```python
from build123d import *

# Parameters (mm, degrees)
F0_R     = 1.092901
F1_DEPTH = 8.89


with BuildPart() as f1:
    # F0 (on Top) → F1 (new body)
    with BuildSketch(Plane.XY):
        with BuildLine():
            Line((-10.186511, 17.824513), (-30.872961, 17.824513))
            Line((-30.872961, 17.824513), (-20.463953, -0.204419))
            Line((-20.463953, -0.204419), (-30.484094, -17.781989))
            Line((-30.484094, -17.781989), (-10.188458, -18.002097))
            Line((-10.188458, -18.002097), (0, -35.649025))
            Line((0, -35.649025), (10.061664, -18.221712))
            Line((10.061664, -18.221712), (31.196423, -18.450921))
            Line((31.196423, -18.450921), (20.562876, -0.033079))
            Line((20.562876, -0.033079), (30.872961, 17.824513))
            Line((30.872961, 17.824513), (10.252791, 17.824513))
            Line((10.252791, 17.824513), (1.863466, 32.35525))
            ThreePointArc((1.863466, 32.35525), (1.860641, 34.526342), (-0.018168, 35.614335))
            ThreePointArc((-0.018168, 35.614335), (-0.0318, 35.614328), (-0.045431, 35.614235))
            ThreePointArc((-0.045431, 35.614235), (-1.914248, 34.515979), (-1.907155, 32.348355))
            Line((-1.907155, 32.348355), (-10.186511, 17.824513))
        make_face()
        Polygon((-7.632454, -18.029818), (7.537469, -18.194337), (0, -31.249616), align=None, mode=Mode.SUBTRACT)
        Polygon((-11.478418, -15.767821), (-26.717751, -15.602549), (-19.193953, -2.404124), align=None, mode=Mode.SUBTRACT)
        Polygon((6.609826, -15.96399), (-6.587783, -15.820861), (-5.245977, -12.983611), (5.37023, -12.983611), align=None, mode=Mode.SUBTRACT)
        Polygon((-10.226373, -13.537018), (-16.653953, -2.404124), (-13.604161, -2.404124), (-8.723036, -10.85848), align=None, mode=Mode.SUBTRACT)
        Polygon((13.711111, -2.218881), (16.760902, -2.218881), (10.064189, -13.817929), (8.537635, -11.179605), align=None, mode=Mode.SUBTRACT)
        Polygon((11.33557, -16.015242), (19.300902, -2.218881), (27.366612, -16.1891), align=None, mode=Mode.SUBTRACT)
        Polygon((-19.20203, 2.009275), (-27.062961, 15.624808), (-11.440459, 15.624808), align=None, mode=Mode.SUBTRACT)
        Polygon((-13.832127, 2.009275), (-16.678082, 2.009275), (-10.170459, 13.425103), (-8.705827, 10.888287), align=None, mode=Mode.SUBTRACT)
        with BuildLine():
            Line((-6.75627, 0.938559), (-7.088266, 1.774853))
            ThreePointArc((-7.088266, 1.774853), (-6.149591, 2.138201), (-5.143329, 2.114348))
            ThreePointArc((-5.143329, 2.114348), (-4.684085, 1.931017), (-4.344395, 1.571676))
            ThreePointArc((-4.344395, 1.571676), (-4.154791, 0.893336), (-4.344395, 0.214996))
            ThreePointArc((-4.344395, 0.214996), (-4.846257, -0.463524), (-5.50511, -0.990941))
            Line((-5.50511, -0.990941), (-4.118282, -0.990941))
            Line((-4.118282, -0.990941), (-4.118282, -1.940617))
            Line((-4.118282, -1.940617), (-7.133126, -1.940617))
            Line((-7.133126, -1.940617), (-7.133126, -1.262277))
            ThreePointArc((-7.133126, -1.262277), (-6.428669, -0.65133), (-5.761372, 0))
            ThreePointArc((-5.761372, 0), (-5.521749, 0.287364), (-5.354368, 0.622))
            ThreePointArc((-5.354368, 0.622), (-5.409921, 1.056041), (-5.79152, 1.270191))
            ThreePointArc((-5.79152, 1.270191), (-6.315562, 1.225589), (-6.75627, 0.938559))
        make_face(mode=Mode.SUBTRACT)
        with BuildLine():
            ThreePointArc((-3.600539, 0.402436), (-3.456783, 1.145183), (-3.035859, 1.773803))
            ThreePointArc((-3.035859, 1.773803), (-2.669777, 2.034358), (-2.238135, 2.159219))
            ThreePointArc((-2.238135, 2.159219), (-1.951313, 2.178043), (-1.664491, 2.159219))
            ThreePointArc((-1.664491, 2.159219), (-1.180923, 1.946357), (-0.821952, 1.558686))
            ThreePointArc((-0.821952, 1.558686), (-0.52188, 0.80677), (-0.454462, 0))
            ThreePointArc((-0.454462, 0), (-0.581823, -0.858949), (-1.010179, -1.614281))
            ThreePointArc((-1.010179, -1.614281), (-1.43468, -1.87918), (-1.924424, -1.981771))
            ThreePointArc((-1.924424, -1.981771), (-2.520232, -1.899523), (-3.044822, -1.605318))
            ThreePointArc((-3.044822, -1.605318), (-3.443663, -0.96578), (-3.582613, -0.224987))
            ThreePointArc((-3.582613, -0.224987), (-3.602765, 0.088404), (-3.600539, 0.402436))
        make_face(mode=Mode.SUBTRACT)
        Polygon((-4.867668, 12.983611), (-6.392563, 15.624808), (6.461138, 15.624808), (4.938996, 12.983611), align=None, mode=Mode.SUBTRACT)
        Polygon((-7.662563, 17.824513), (-0.015805, 31.238637), (7.728844, 17.824513), align=None, mode=Mode.SUBTRACT)
        with Locations((-0.023831, 33.438342)):
            Circle(F0_R, mode=Mode.SUBTRACT)
        Polygon((0.406004, 0.787853), (0.235703, 1.612465), (1.382991, 2.10544), (2.315162, 2.10544), (2.315162, -1.919029), (1.221654, -1.919029), (1.221654, 1.11949), align=None, mode=Mode.SUBTRACT)
        with BuildLine():
            ThreePointArc((6.263092, 1.305151), (5.667589, 1.281478), (5.09484, 1.116724))
            ThreePointArc((5.09484, 1.116724), (4.817232, 0.89738), (4.657688, 0.581589))
            ThreePointArc((4.657688, 0.581589), (5.038025, 0.762238), (5.456621, 0.807702))
            ThreePointArc((5.456621, 0.807702), (5.84702, 0.774991), (6.187721, 0.581589))
            ThreePointArc((6.187721, 0.581589), (6.553589, 0.245128), (6.715319, -0.224882))
            ThreePointArc((6.715319, -0.224882), (6.710022, -0.667762), (6.609799, -1.099186))
            ThreePointArc((6.609799, -1.099186), (6.363355, -1.487281), (6.00683, -1.777526))
            ThreePointArc((6.00683, -1.777526), (5.523997, -1.951951), (5.011932, -1.988565))
            ThreePointArc((5.011932, -1.988565), (4.415764, -1.838341), (3.919051, -1.476042))
            ThreePointArc((3.919051, -1.476042), (3.611747, -0.926696), (3.496973, -0.30779))
            ThreePointArc((3.496973, -0.30779), (3.537223, 0.33579), (3.753235, 0.94337))
            ThreePointArc((3.753235, 0.94337), (4.096734, 1.436393), (4.567243, 1.810138))
            ThreePointArc((4.567243, 1.810138), (5.106743, 2.061392), (5.694663, 2.153803))
            ThreePointArc((5.694663, 2.153803), (5.728652, 2.154074), (5.762642, 2.153803))
            Line((5.762642, 2.153803), (6.268268, 2.153803))
            Line((6.268268, 2.153803), (6.263092, 1.305151))
        make_face(mode=Mode.SUBTRACT)
        Polygon((8.786237, 10.749013), (10.278659, 13.408103), (16.768929, 2.166626), (13.74128, 2.166626), align=None, mode=Mode.SUBTRACT)
        Polygon((11.522791, 15.624808), (27.062961, 15.624808), (19.292876, 2.166626), align=None, mode=Mode.SUBTRACT)
    extrude(amount=F1_DEPTH)


solid = f1.part
```
The model under review builds one solid part; all positions refer to its coordinate system, in mm. A direction names the side the tool comes from. Give positions to 0.01 mm unless a question says otherwise; leave off trailing zeros. Loops run counter-clockwise (first coordinate to the right, second up) from the corner with the lowest first, then second, coordinate; pieces in that order, holes last. Notation, with made-up numbers: (85.25, 61.25) -> (98.25, 61.25) arc R12 cw to (98.25, 74.25) -> close; hole circle Ø2 at (-37.75, -16.75). An arc over 180 degrees is marked (long way). Use CSV: the item, a comma, the result in double quotes.
1. Consider section C-C, the plane x = -15. Write out the cut boundary in (y, z), then the cut area to 3 significant figures.
Result:
outline,"(-17.95, 0) -> (-15.73, 0) -> (-15.73, 8.89) -> (-17.95, 8.89) -> close; (-9.67, 0) -> (-5.27, 0) -> (-5.27, 8.89) -> (-9.67, 8.89) -> close; (-2.4, 0) -> (2.01, 0) -> (2.01, 8.89) -> (-2.4, 8.89) -> close; (4.95, 0) -> (9.38, 0) -> (9.38, 8.89) -> (4.95, 8.89) -> close; (15.62, 0) -> (17.82, 0) -> (17.82, 8.89) -> (15.62, 8.89) -> close"
area,"157 mm²"
2. Consider section A-A, the plane x = 23.5. Write out the cut boundary in (y, z).
Result:
outline,"(-18.37, 0) -> (-16.15, 0) -> (-16.15, 8.89) -> (-18.37, 8.89) -> close; (-9.49, 0) -> (-5.12, 0) -> (-5.12, 8.89) -> (-9.49, 8.89) -> close; (5.05, 0) -> (9.45, 0) -> (9.45, 8.89) -> (5.05, 8.89) -> close; (15.62, 0) -> (17.82, 0) -> (17.82, 8.89) -> (15.62, 8.89) -> close"
3. Consider section D-D, the plane y = -25.5. Write out the cut boundary in (x, z), then the cut area to 3 significant figures.
Result:
outline,"(-5.86, 0) -> (-3.32, 0) -> (-3.32, 8.89) -> (-5.86, 8.89) -> close; (3.32, 0) -> (5.86, 0) -> (5.86, 8.89) -> (3.32, 8.89) -> close"
area,"45.2 mm²"
4. For P1, Ø2.5, axis at x = -22.5, z = 3.5, coming from the -Y side; P2, Ø2.5, axis at y = -0.5, z = 4.5, coming from the +X side; P3, Ø0.5, axis at x = 2, z = 5.5, coming from the -Y side, all flat-tipped, find the tip position at first contact; note any pin that passes through.
Result:
P1,"stops at y = -17.88"
P2,"stops at x = 21.55"
P3,"stops at y = -32.62"
5. Consider section B-B, the plane y = 3. Write out the cut boundary in (x, z).
Result:
outline,"(-22.31, 0) -> (-19.77, 0) -> (-19.77, 8.89) -> (-22.31, 8.89) -> close; (-18.64, 0) -> (-16.11, 0) -> (-16.11, 8.89) -> (-18.64, 8.89) -> close; (-13.26, 0) -> (13.26, 0) -> (13.26, 8.89) -> (-13.26, 8.89) -> close; (16.29, 0) -> (18.81, 0) -> (18.81, 8.89) -> (16.29, 8.89) -> close; (19.77, 0) -> (22.31, 0) -> (22.31, 8.89) -> (19.77, 8.89) -> close"
6. The part is to be moulded in two halves that separate along Y. For faces 3 (the face through (4.96, -27.06, 4.38)), 4 (the face through (9.3, -12.5, 4.4)), say which applies: +Y half, -Y half, draft (parallel to the pull), parting line (faces both ways), or undercut.
Result:
face 3,"-Y half"
face 4,"undercut"
7. Machinability: for faces 1 (the face through (0, 12.984, 4)), 2 (the face through (25.646, 8.771, 4.383)), which of the approach directions +Z, -Z, +X, -X, +Y, -Y give a long, thin tool a straight path to every point of the face, cutting with its end or side? Answer none if there is none.
Result:
face 1,"+Z, -Z"
face 2,"+Z, -Z, +X"
8. To check wall thickness, follow probe 1 along Y at (x, z) = (4.5, 5.5); probe 2 along X at (y, z) = (6, 2); probe 3 along X at (y, z) = (-14.5, 2.75). State the ranges of each line that lie inside material, in increasing order. Write a range as from..to.
Result:
probe 1,"y = -27.85..-23.46, -18.16..-15.94, -12.98..-1.87, 1.77..12.98, 15.62..17.82, 23.42..27.79"
probe 2,"x = -24.05..-21.51, -16.93..-14.4, -11.53..11.53, 14.56..17.08, 21.51..24.05"
probe 3,"x = -28.61..-26.09, -12.21..-5.96, 6..12.21, 26.39..28.92"
